```python
from build123d import *

# Parameters (mm, degrees)
EXTRUSION1_DEPTH        = 20
ENL_V_MAT_EXTRU_1_DEPTH = 136.838138974


with BuildPart() as part:
    # Esquisse1 → Extrusion1 (new body)
    with BuildSketch(Plane.XY):
        with BuildLine():
            Line((75.5, 95), (-75.5, 95))
            ThreePointArc((-75.5, 95), (-75.853553391, 94.853553391), (-76, 94.5))
            Line((-76, 94.5), (-76, 1.5))
            ThreePointArc((-76, 1.5), (-76.439339828, 0.439339828), (-77.5, 0))
            Line((-77.5, 0), (-94, 0))
            Line((-94, 0), (-94, 1))
            Line((-94, 1), (-77.5, 1))
            ThreePointArc((-77.5, 1), (-77.146446609, 1.146446609), (-77, 1.5))
            Line((-77, 1.5), (-77, 94.5))
            ThreePointArc((-77, 94.5), (-76.560660172, 95.560660172), (-75.5, 96))
            Line((-75.5, 96), (75.5, 96))
            ThreePointArc((75.5, 96), (76.560660172, 95.560660172), (77, 94.5))
            Line((77, 94.5), (77, 1.5))
            ThreePointArc((77, 1.5), (77.146446609, 1.146446609), (77.5, 1))
            Line((77.5, 1), (94, 1))
            Line((94, 1), (94, 0))
            Line((94, 0), (77.5, 0))
            ThreePointArc((77.5, 0), (76.439339828, 0.439339828), (76, 1.5))
            Line((76, 1.5), (76, 94.5))
            ThreePointArc((76, 94.5), (75.853553391, 94.853553391), (75.5, 95))
        make_face()
    extrude(amount=EXTRUSION1_DEPTH)

    # Esquisse2 → Enlèv. mat.-Extru.1 (cut, through all)
    with BuildSketch(Plane.XZ):
        with BuildLine():
            Line((-89.5, 12.5), (-82.5, 12.5))
            ThreePointArc((-82.5, 12.5), (-80, 10), (-82.5, 7.5))
            Line((-82.5, 7.5), (-89.5, 7.5))
            ThreePointArc((-89.5, 7.5), (-92, 10), (-89.5, 12.5))
        make_face()
        with BuildLine():
            Line((89.5, 7.5), (82.5, 7.5))
            ThreePointArc((82.5, 7.5), (80, 10), (82.5, 12.5))
            Line((82.5, 12.5), (89.5, 12.5))
            ThreePointArc((89.5, 12.5), (92, 10), (89.5, 7.5))
        make_face()
    extrude(amount=-ENL_V_MAT_EXTRU_1_DEPTH, mode=Mode.SUBTRACT)


solid = part.part
```
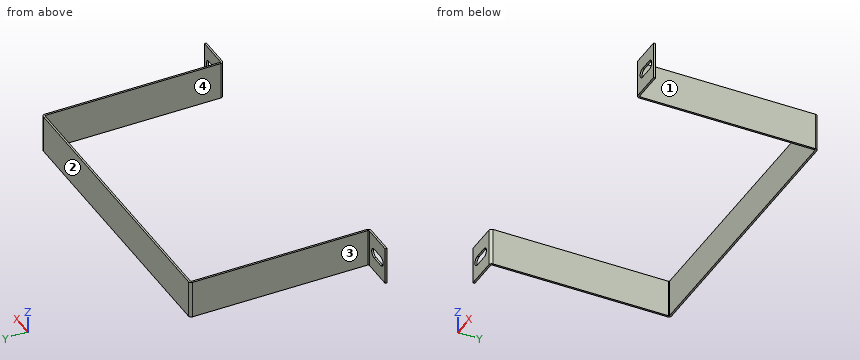
Design review of the part built by this model. Coordinates are the model's own, in mm. Face numbers are marked on the shaded views. Coordinates: 2 decimals unless noted, no trailing zeros. Loops run counter-clockwise (first coordinate to the right, second up) from the corner with the lowest first, then second, coordinate; pieces in that order, holes last. Notation, with made-up numbers: (-16.75, -32.75) - (21.25, -32.75) arc R22 cw to (21.25, -3.75) - close; hole circle Ø1 at (19, 86.5). An arc over 180 degrees is marked (long way). Use CSV: the item, a comma, the result in double quotes. Start each with the question number.
1) Consider section C-C on x = 43.5. Write out the cut boundary in (y, z), then the cut area to 3 significant figures.
2) For pin 1 Ø5 at (x, z) = (83.5, 13) entering from +Y; pin 2 Ø6 at (y, z) = (56, 7.5) entering from +X; pin 3 Ø10 at (x, z) = (31, 11.5) entering from -Y, all flat-tipped, find the tip position at first contact; note any pin that passes through.
3) Wall thickness on L1, parallel to X at y = 48.5, z = 17.25; L2, parallel to Y at x = 62, z = 1.5; L3, parallel to Y at x = 81, z = 4.5: over which ranges is each line inside the solid? List them lowest first. Write a range as from..to.
4) The part is to be moulded in two halves that separate along X. For the marked faces 1, 2, 3 and 4, say which applies: +X half, -X half, draft (parallel to the pull), parting line (faces both ways), or undercut.
5) Consider section B-B on z = 9.5. Write out the cut boundary in (x, y), then the cut area to 3 significant figures.
6) Consider section A-A on y = 62.5. Write out the cut boundary in (x, z), then the cut area to 3 significant figures.
Geometry says:
1,outline,"(95, 0) - (96, 0) - (96, 20) - (95, 20) - close"
1,area,"20.0 mm^2"
2,pin 1,"y = 1"
2,pin 2,"x = 77"
2,pin 3,"y = 95"
3,L1,"-77..-76, 76..77"
3,L2,"95..96"
3,L3,"0..1"
4,face 1,"+X half"
4,face 2,"draft"
4,face 3,"-X half"
4,face 4,"undercut"
5,outline,"(-94, 0) - (-91.95, 0) - (-91.95, 1) - (-94, 1) - close; (-80.05, 0) - (-77.5, 0) arc R1.5 ccw to (-76, 1.5) - (-76, 94.5) arc R0.5 cw to (-75.5, 95) - (75.5, 95) arc R0.5 cw to (76, 94.5) - (76, 1.5) arc R1.5 ccw to (77.5, 0) - (80.05, 0) - (80.05, 1) - (77.5, 1) arc R0.5 cw to (77, 1.5) - (77, 94.5) arc R1.5 ccw to (75.5, 96) - (-75.5, 96) arc R1.5 ccw to (-77, 94.5) - (-77, 1.5) arc R0.5 cw to (-77.5, 1) - (-80.05, 1) - close; (91.95, 0) - (94, 0) - (94, 1) - (91.95, 1) - close"
5,area,"352 mm^2"
6,outline,"(-77, 0) - (-76, 0) - (-76, 20) - (-77, 20) - close; (76, 0) - (77, 0) - (77, 20) - (76, 20) - close"
6,area,"40.0 mm^2"
